For this review, take the finished solid that the model builds, in its own axes (mm). A direction names the side the tool comes from. Coordinates: 2 decimals unless noted, no trailing zeros. Loops run counter-clockwise (first coordinate to the right, second up) from the corner with the lowest first, then second, coordinate; pieces in that order, holes last. Notation, with made-up numbers: (-26, 59.25) - (-7, 59.25) arc R36 ccw to (-7, 98.25) - close; hole circle Ø2 at (2.5, 35). An arc over 180 degrees is marked (long way). Use one line per item in the form item = value. Start each with the question number.
1. Add section C-C on x = 73. Give the boundary of the cut face in (y, z).
2. Machinability: for faces 1 (the face through (-1, 0, -1)), 2 (the face through (73, 2.6, -53)), 3 (the face through (50, 5, -52)), 4 (the face through (-6, 3, 34)), which of the approach directions +Z, -Z, +X, -X, +Y, -Y give a long, thin tool a straight path to every point of the face, cutting with its end or side? Answer none if there is none.
3. For pin 1 Ø1.8 at (x, z) = (-27, 19.95) entering from -Y, flat-tipped, find the tip position at first contact; note if it passes through.
4. Draft analysis for pull direction Z (two halves, no side actions). For faces 5 (the face through (54, 6, -49)), 6 (the face through (83, 3, 64)), 7 (the face through (48, 3, 34)), state which applies: +Z half, -Z half, draft (parallel to the pull), parting line (faces both ways), or undercut.
5. To check wall thickness, follow probe 1 along X at (y, z) = (3.1, 11.95); probe 2 along X at (y, z) = (1.05, 38.5); probe 3 along X at (y, z) = (1.8, 53). State the ranges of each line that lie inside material, in increasing order.
6. Add section B-B on y = 5. Count the separate pieces of the cut face and the enclosed holes in it, and give its area (3 significant figures).
7. Add section A-A on z = 25. Give the boundary of the cut face in (x, y), and give its area (3 significant figures).
8. Add section D-D on z = 53. Give the boundary of the cut face in (x, y).
```python
from build123d import *

# Parameters (mm, degrees)
SKETCH1_W               = 170
SKETCH1_H               = 130
BOSS_EXTRUDE1_DEPTH     = 6
SKETCH2_R               = 1
SKETCH2_R_2             = 2
SKETCH2_W               = 12
SKETCH2_H               = 22.4
CUT_EXTRUDE1_DEPTH      = 10
LPATTERN1_COUNT         = 5
LPATTERN1_PITCH         = 27
SKETCH8_W               = 25
SKETCH8_H               = 25
CUT_EXTRUDE5_DEPTH      = 108.172757733
FILLET2_R               = 5
SKETCH10_R              = 9
CUT_EXTRUDE6_DEPTH      = 2.6
MIRROR2_COPY_1_SKETCH_R = 9
MIRROR2_COPY_1_DEPTH    = 2.6
CUT_EXTRUDE7_DEPTH      = 3


with BuildPart() as part:
    # Sketch1 → Boss-Extrude1 (new body)
    with BuildSketch(Plane(origin=(0, 0, 0), x_dir=(1, 0, 0), z_dir=(0, 1, 0))):
        Rectangle(SKETCH1_W, SKETCH1_H)
    extrude(amount=BOSS_EXTRUDE1_DEPTH)

    # Sketch2 → Cut-Extrude1 (cut)
    with BuildSketch(Plane(origin=(0, 6, 0), x_dir=(1, 0, 0), z_dir=(0, 1, 0))):
        with Locations(Location((-54, -19.95, 0), (0, 0, 270))):
            Circle(SKETCH2_R)
        with Locations(Location((-54, -47.65, 0), (0, 0, 270))):
            Circle(SKETCH2_R)
        with Locations(Location((-54, -11.95, 0), (0, 0, 270))):
            Circle(SKETCH2_R_2)
        with Locations((-54, -33.8)):
            Rectangle(SKETCH2_W, SKETCH2_H)
    cut_extrude1 = extrude(amount=-CUT_EXTRUDE1_DEPTH, mode=Mode.SUBTRACT)

    # LPattern1: Cut-Extrude1 ×5
    with Locations(*[(i * LPATTERN1_PITCH, 0, 0) for i in range(1, LPATTERN1_COUNT)]):
        add(cut_extrude1, mode=Mode.SUBTRACT)

    # Sketch8 → Cut-Extrude5 (cut, through all)
    with BuildSketch(Plane(origin=(0, 6, 0), x_dir=(1, 0, 0), z_dir=(0, 1, 0))):
        with Locations((54.5, 23.55)):
            Rectangle(SKETCH8_W, SKETCH8_H)
    extrude(amount=-CUT_EXTRUDE5_DEPTH, mode=Mode.SUBTRACT)

    # Fillet2
    fillet2_edges = [part.edges().sort_by_distance(p)[0] for p in [
        (85, 3, 65),
        (-85, 3, 65),
    ]]
    fillet(fillet2_edges, radius=FILLET2_R)

    # Sketch10 → Cut-Extrude6 (cut)
    with BuildSketch(Plane.XZ):
        with Locations(Location((-73, 53, 0), (0, 0, 270))):
            Circle(SKETCH10_R)
    cut_extrude6 = extrude(amount=-CUT_EXTRUDE6_DEPTH, mode=Mode.SUBTRACT)

    # Mirror1: Cut-Extrude6 across plane
    add(cut_extrude6.mirror(Plane(origin=(0, 0, 0), x_dir=(0, 0, 1), z_dir=(1, 0, 0))), mode=Mode.SUBTRACT)

    # Mirror2: Cut-Extrude6 across plane
    add(cut_extrude6.mirror(Plane.XY), mode=Mode.SUBTRACT)

    # Mirror2 copy 1 sketch → Mirror2 copy 1 (cut)
    with BuildSketch(Plane(origin=(0, 0, 0), x_dir=(-1, 0, 0), z_dir=(0, -1, 0))):
        with Locations(Location((-73, 53, 0), (0, 0, 270))):
            Circle(MIRROR2_COPY_1_SKETCH_R)
    extrude(amount=-MIRROR2_COPY_1_DEPTH, mode=Mode.SUBTRACT)

    # Sketch11 → Cut-Extrude7 (cut)
    with BuildSketch(Plane(origin=(0, 6, 0), x_dir=(1, 0, 0), z_dir=(0, 1, 0))):
        Polygon((45.897368421, 40.869502872), (50.042105263, 49.063376227), (46.292105263, 56.066871293), (61.489473684, 56.066871293), (57.936842105, 49.072627872), (62.278947368, 40.869502872), align=None)
        Polygon((47.932730263, 42.053713398), (53.989473684, 42.053713398), (51.765995066, 45.856139385), (52.55546875, 47.065020964), (55.525246711, 42.053713398), (60.17265625, 42.053713398), (56.357894737, 49.069543991), (59.438692434, 54.882660767), (54.686430921, 54.882660767), (56.191365132, 52.366213398), (55.380304276, 51.151164056), (53.088980263, 54.882660767), (48.404564145, 54.882660767), (51.621052632, 49.075711754), align=None, mode=Mode.SUBTRACT)
    extrude(amount=-CUT_EXTRUDE7_DEPTH, mode=Mode.SUBTRACT)


solid = part.part
```
Conclusion:
q1.outline = (0, -65) - (6, -65) - (6, 65) - (0, 65) - (0, 62) - (2.6, 62) - (2.6, 44) - (0, 44) - (0, -44) - (2.6, -44) - (2.6, -62) - (0, -62) - close
q2.face_1 = +Z, -Z, +X, -X, -Y
q2.face_2 = -Y
q2.face_3 = +Y
q2.face_4 = +Y, -Y
q3.pin_1 = through
q4.face_5 = draft
q4.face_6 = +Z half
q4.face_7 = undercut
q5.probe_1 = -85 to -56, -52 to -29, -25 to -2, 2 to 25, 29 to 52, 56 to 85
q5.probe_2 = -85 to -60, -48 to -33, -21 to -6, 6 to 21, 33 to 48, 60 to 85
q5.probe_3 = -85 to -82, -64 to 64, 82 to 85
q6.separate_pieces = 2
q6.enclosed_holes = 22
q6.area = 19,900 mm^2
q7.outline = (-85, 0) - (-60, 0) - (-60, 6) - (-85, 6) - close; (-48, 0) - (-33, 0) - (-33, 6) - (-48, 6) - close; (-21, 0) - (-6, 0) - (-6, 6) - (-21, 6) - close; (6, 0) - (21, 0) - (21, 6) - (6, 6) - close; (33, 0) - (48, 0) - (48, 6) - (33, 6) - close; (60, 0) - (85, 0) - (85, 6) - (60, 6) - close
q7.area = 660 mm^2
q8.outline = (-85, 0) - (-82, 0) - (-82, 2.6) - (-64, 2.6) - (-64, 0) - (64, 0) - (64, 2.6) - (82, 2.6) - (82, 0) - (85, 0) - (85, 6) - (-85, 6) - close
